The drawing under review shows one solid part. Ordinate dimensions are in mm from its lowest x, y, z. A direction names the side the tool comes from. Round coordinates to 2 decimals unless told otherwise and drop trailing zeros. Order: outer loops, then holes, each group sorted by start corner. A loop starts at its lowest first (then second) coordinate and runs counter-clockwise, first axis right, second up. Notation, with made-up numbers: M 13,-32 L 32,-32 A13 cw 32,-12 Z; hole C 28,51 d10. An arc over 180 degrees is marked long. Use a Markdown table: item, result.
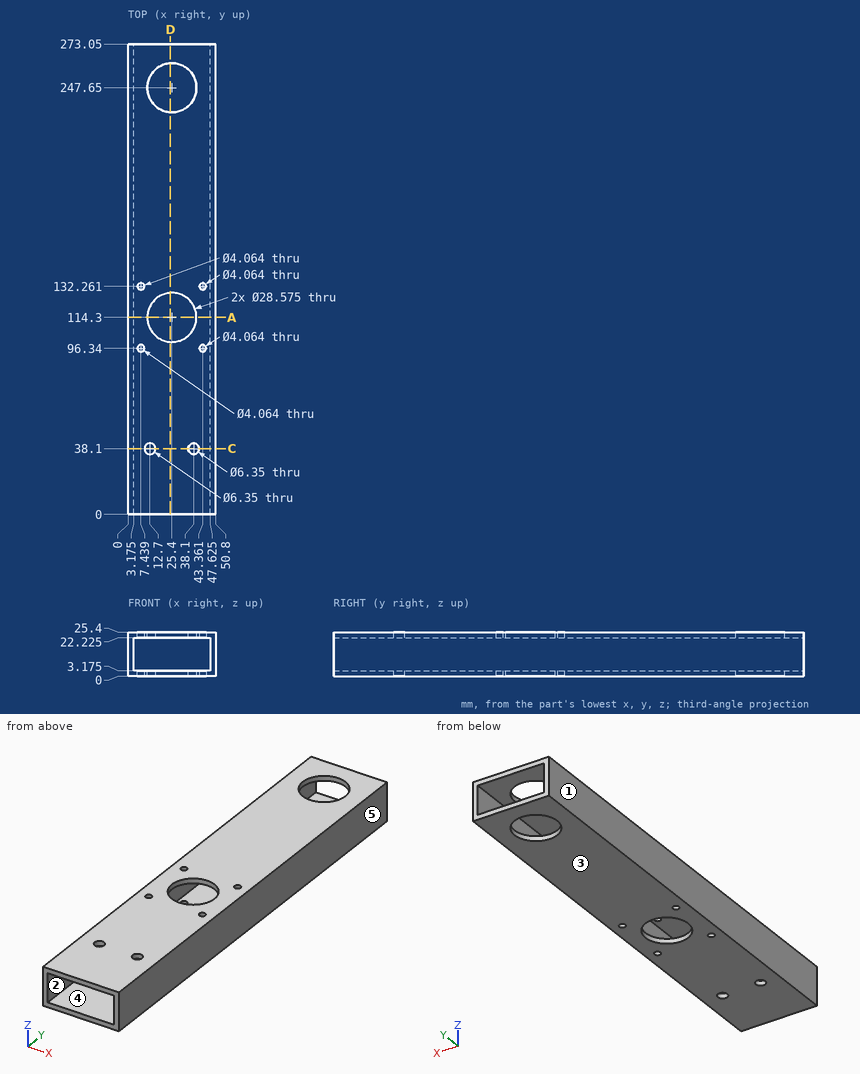
Q1. Add section A-A (y = 114.3). Write out the cut boundary in (x, z) (1 decimal).
Determined:
| item | result |
|---|---|
| outline | M 0,0 L 11.1,0 L 11.1,3.2 L 3.2,3.2 L 3.2,22.2 L 11.1,22.2 L 11.1,25.4 L 0,25.4 Z; M 39.7,0 L 50.8,0 L 50.8,25.4 L 39.7,25.4 L 39.7,22.2 L 47.6,22.2 L 47.6,3.2 L 39.7,3.2 Z |
Q2. Draft analysis for pull direction X (two halves, no side actions). For the marked faces 1, 2 and 3, state which applies: pulls with the +X half, pulls with the -X half, needs draft (parallel to the pull), parting line crosses it, or undercut.
Determined:
| item | result |
|---|---|
| face 1 | pulls with the -X half |
| face 2 | undercut |
| face 3 | needs draft |
Q3. Add section C-C (y = 38.1). Write out the cut boundary in (x, z) (1 decimal).
Determined:
| item | result |
|---|---|
| outline | M 0,0 L 9.5,0 L 9.5,3.2 L 3.2,3.2 L 3.2,22.2 L 9.5,22.2 L 9.5,25.4 L 0,25.4 Z; M 15.9,0 L 34.9,0 L 34.9,3.2 L 15.9,3.2 Z; M 15.9,22.2 L 34.9,22.2 L 34.9,25.4 L 15.9,25.4 Z; M 41.3,0 L 50.8,0 L 50.8,25.4 L 41.3,25.4 L 41.3,22.2 L 47.6,22.2 L 47.6,3.2 L 41.3,3.2 Z |
Q4. Clearance check with a flat-ended pin moving along its axis: pin 1 (5 mm diameter, centred on x = 38.1, y = 38.1, fed in from -Z). State where the tip first meets the part, or that it passes through.
Determined:
| item | result |
|---|---|
| pin 1 | passes through |
Q5. Machinability: for the marked faces 4 and 5, which of the approach directions +Z, -Z, +X, -X, +Y, -Y give a long, thin tool a straight path to every point of the face, cutting with its end or side? Answer none if there is none.
Determined:
| item | result |
|---|---|
| face 4 | +Y, -Y |
| face 5 | +Z, -Z, +X, +Y, -Y |
Q6. Add section D-D (x = 24.5). Give the number of separate pieces and of enclosed holes in the cut face, then the cut area to 3 significant figures.
Determined:
| item | result |
|---|---|
| separate pieces | 6 |
| enclosed holes | 0 |
| area | 1,370 mm^2 |
Q7. Wall thickness on line 1 along Z through (x, y) = (36, 229) (1 decimal); line 2 along X through (y, z) = (185, 9.5) (1 decimal); line 3 along X through (y, z) = (251.5, 24): over which ranges is each line inside the solid? List them lowest first. Write a range as [from, to].
Determined:
| item | result |
|---|---|
| line 1 | z = [0, 3.2], [22.2, 25.4] |
| line 2 | x = [0, 3.2], [47.6, 50.8] |
| line 3 | x = [0, 11.64], [39.16, 50.8] |
